```python
from build123d import *

# Parameters (mm, degrees)
BOSS_EXTRUDE1_DEPTH     = 7.5
BOSS_EXTRUDE2_START     = -7.5
SKETCH1_3_W             = 46
SKETCH1_3_H             = 36.5
BOSS_EXTRUDE2_DEPTH     = 5
BOSS_EXTRUDE3_DEPTH     = 2.5
BOSS_EXTRUDE4_DEPTH     = 5
CUT_EXTRUDE1_START      = -5
CUT_EXTRUDE1_DEPTH      = 3
M2_5_CLEARANCE_HOLE1_D  = 2.9
MIRROR1_START           = -16.25
MIRROR1_DEPTH           = 3
MIRROR1_START_2         = -18.25
MIRROR1_2_DEPTH         = 5
MIRROR1_3_OUTLINE_R     = 1.45
MIRROR1_3_DEPTH         = 2
MIRROR1_START_3         = 23
MIRROR1_4_DEPTH         = 2.5
CUT_EXTRUDE2_DEPTH      = 37.094632565
CUT_EXTRUDE2_DEPTH_BACK = 37.094632565
SKETCH10_W              = 15
SKETCH10_H              = 21
CHAMFER1_SIZE           = 5
FILLET1_R               = 1
FILLET2_R               = 1
FILLET6_R               = 1
FILLET7_R               = 1
FILLET8_R               = 1


with BuildPart() as part:
    # Sketch1 → Boss-Extrude1 (new, symmetric)
    with BuildSketch(Plane(origin=(0, 0, 0), x_dir=(1, 0, 0), z_dir=(0, 1, 0))):
        Polygon((23, -18.25), (-23, -18.25), (-23, 18.25), (-25.5, 18.25), (-25.5, -20.75), (25.5, -20.75), (25.5, 18.25), (23, 18.25), align=None)
    extrude(amount=BOSS_EXTRUDE1_DEPTH, both=True)

    # Sketch1<3> → Boss-Extrude2 (add)
    with BuildSketch(Plane(origin=(0, 0, 0), x_dir=(1, 0, 0), z_dir=(0, 1, 0)).offset(BOSS_EXTRUDE2_START)):
        Rectangle(SKETCH1_3_W, SKETCH1_3_H)
    extrude(amount=BOSS_EXTRUDE2_DEPTH)

    # Sketch5 → Boss-Extrude3 (add)
    with BuildSketch(Plane(origin=(-25.5, 32.25, 0), x_dir=(0, 1, 0), z_dir=(-1, 0, 0))):
        Polygon((-47.15, 18.25), (-39.75, 18.25), (-39.75, -20.75), (-47.15, 13.25), align=None)
    extrude(amount=-BOSS_EXTRUDE3_DEPTH)

    # Sketch6 → Boss-Extrude4 (add)
    with BuildSketch(Plane(origin=(0, 0, -18.25), x_dir=(-1, 0, 0), z_dir=(0, 0, -1))):
        Polygon((-12, -10.3), (-14.266838493, -10.3), (-15.883419246, -13.1), (-19.116580754, -13.1), (-20.733161507, -10.3), (-19.116580754, -7.5), (-23, -7.5), (-23, -14.9), (-12, -14.9), align=None)
        Polygon((23, -7.5), (12, -7.5), (12, -10.3), (12, -14.9), (23, -14.9), align=None)
    extrude(amount=-BOSS_EXTRUDE4_DEPTH)

    # Sketch6<3> → Cut-Extrude1 (cut)
    with BuildSketch(Plane(origin=(0, 0, -18.25), x_dir=(-1, 0, 0), z_dir=(0, 0, -1)).offset(CUT_EXTRUDE1_START)):
        Polygon((19.0011107, -7.7), (15.9988893, -7.7), (14.4977786, -10.3), (15.9988893, -12.9), (19.0011107, -12.9), (20.5022214, -10.3), align=None)
    extrude(amount=CUT_EXTRUDE1_DEPTH, mode=Mode.SUBTRACT)

    # M2.5 Clearance Hole1 (through all)
    with Locations(Plane.XY.offset(-16.25)):
        with Locations((-17.5, -10.3), (17.5, -10.3)):
            Hole(M2_5_CLEARANCE_HOLE1_D / 2)

    # Mirror1: read off the stored shape, not the designer's step
    # Mirror1 outline → Mirror1 (cut)
    with BuildSketch(Plane.XY.offset(MIRROR1_START)):
        Polygon((-14.266838493, -10.3), (-15.883419246, -7.5), (-19.116580754, -7.5), (-20.733161507, -10.3), (-19.116580754, -13.1), (-15.883419246, -13.1), align=None)
        Polygon((-15.9988893, -12.9), (-19.0011107, -12.9), (-20.5022214, -10.3), (-19.0011107, -7.7), (-15.9988893, -7.7), (-14.4977786, -10.3), align=None, mode=Mode.SUBTRACT)
    extrude(amount=MIRROR1_DEPTH, mode=Mode.SUBTRACT)

    # Mirror1 2 outline → Mirror1 2 (add)
    with BuildSketch(Plane.XY.offset(MIRROR1_START_2)):
        Polygon((20.733161507, -10.3), (19.116580754, -7.5), (12, -7.5), (12, -10.3), (14.266838493, -10.3), (15.883419246, -13.1), (19.116580754, -13.1), align=None)
        Polygon((15.9988893, -7.7), (19.0011107, -7.7), (20.5022214, -10.3), (19.0011107, -12.9), (15.9988893, -12.9), (14.4977786, -10.3), align=None, mode=Mode.SUBTRACT)
    extrude(amount=MIRROR1_2_DEPTH)

    # Mirror1 3 outline → Mirror1 3 (add)
    with BuildSketch(Plane.XY.offset(MIRROR1_START_2)):
        Polygon((20.5022214, -10.3), (19.0011107, -7.7), (15.9988893, -7.7), (14.4977786, -10.3), (15.9988893, -12.9), (19.0011107, -12.9), align=None)
        with Locations((17.5, -10.3)):
            Circle(MIRROR1_3_OUTLINE_R, mode=Mode.SUBTRACT)
    extrude(amount=MIRROR1_3_DEPTH)

    # Mirror1 4 outline → Mirror1 4 (add)
    with BuildSketch(Plane.YZ.offset(MIRROR1_START_3)):
        Polygon((-14.9, -13.25), (-14.9, -18.25), (-7.5, -18.25), (-7.5, 20.75), align=None)
    extrude(amount=MIRROR1_4_DEPTH)

    # Sketch10 → Cut-Extrude2 (cut, two sides: drawn at the far end of the back side and taken through both)
    with BuildSketch(Plane(origin=(0, 0, 0), x_dir=(1, 0, 0), z_dir=(0, 1, 0)).offset(-CUT_EXTRUDE2_DEPTH_BACK)):
        with Locations((-15.5, 0)):
            Rectangle(SKETCH10_W, SKETCH10_H)
    extrude(amount=CUT_EXTRUDE2_DEPTH + CUT_EXTRUDE2_DEPTH_BACK, mode=Mode.SUBTRACT)

    # Chamfer1
    chamfer1_edges = [part.edges().sort_by_distance(p)[0] for p in [
        (-8, -5, -10.5),
        (-8, -5, 10.5),
    ]]
    chamfer(chamfer1_edges, length=CHAMFER1_SIZE)

    # Fillet1
    fillet1_edges = [part.edges().sort_by_distance(p)[0] for p in [
        (23, 7.5, 0),
        (-23, 2.5, -18.25),
        (-23, 2.5, 18.25),
        (23, 2.5, 18.25),
        (23, 2.5, -18.25),
        (0, 7.5, 18.25),
        (-23, 7.5, 0),
        (-23, -2.5, -14.375),
        (-18, -2.5, -10.5),
        (-23, -5, -10.5),
        (-23, -5, 10.5),
        (-8, -2.5, 0),
        (-18, -2.5, 10.5),
        (-23, -2.5, 14.375),
        (-10.5, -2.5, 8),
        (-10.5, -2.5, -8),
        (0, -2.5, -18.25),
        (0, -2.5, 18.25),
        (23, -2.5, 0),
    ]]
    fillet(fillet1_edges, radius=FILLET1_R)

    # Fillet2
    fillet2_edges = [part.edges().sort_by_distance(p)[0] for p in [
        (25.5, -14.9, -15.75),
        (25.5, -11.2, 3.75),
        (25.5, 0, 20.75),
        (-25.5, 0, 20.75),
        (-25.5, -3.7, -18.25),
        (25.5, -3.7, -18.25),
        (-25.5, 7.5, 1.25),
        (-25.5, -14.9, -15.75),
        (-25.5, -11.2, 3.75),
        (25.5, 7.5, 1.25),
    ]]
    fillet(fillet2_edges, radius=FILLET2_R)

    # Fillet6
    fillet6_edges = [part.edges().sort_by_distance(p)[0] for p in [
        (-12, -14.9, -15.75),
        (12, -14.9, -15.75),
        (12, -11.2, -13.25),
    ]]
    fillet(fillet6_edges, radius=FILLET6_R)

    # Fillet7
    # the kernel refuses this fillet: 1 mm, written as the material it takes off along each edge
    with BuildSketch(Plane(origin=(24.5, 6.5, 19.75), x_dir=(0, 0, 1), z_dir=(0, 1, 0))) as fillet7_piece_1_section:
        Polygon((0, 0), (FILLET7_R, 0), (FILLET7_R, FILLET7_R), (0, FILLET7_R), align=None)
    fillet7_piece_1 = extrude(amount=FILLET7_R, mode=Mode.PRIVATE)
    fillet7_piece_1 = fillet7_piece_1 - Plane(origin=(24.5, 6.5, 19.75), x_dir=(-0.7071067811865476, 0, -0.7071067811865475), z_dir=(0, 1, 0)) * Sphere(FILLET7_R, mode=Mode.PRIVATE)
    add(fillet7_piece_1, mode=Mode.SUBTRACT)
    with BuildSketch(Plane(origin=(-24.5, 6.5, 19.75), x_dir=(0, 0, 1), z_dir=(0, 1, 0))) as fillet7_piece_2_section:
        Polygon((0, 0), (FILLET7_R, 0), (FILLET7_R, -FILLET7_R), (0, -FILLET7_R), align=None)
    fillet7_piece_2 = extrude(amount=FILLET7_R, mode=Mode.PRIVATE)
    fillet7_piece_2 = fillet7_piece_2 - Plane(origin=(-24.5, 6.5, 19.75), x_dir=(0.7071067811865475, 0, -0.7071067811865475), z_dir=(0, 1, 0)) * Sphere(FILLET7_R, mode=Mode.PRIVATE)
    add(fillet7_piece_2, mode=Mode.SUBTRACT)
    with BuildSketch(Plane(origin=(-24.5, 7.5, 20.75), x_dir=(0, 0, -1), z_dir=(1, 0, 0))) as fillet7_piece_3:
        with BuildLine():
            CenterArc((FILLET7_R, -FILLET7_R), FILLET7_R, 90, 90)
            Line((0, -FILLET7_R), (0, 0))
            Line((0, 0), (FILLET7_R, 0))
        make_face()
    extrude(amount=49, mode=Mode.SUBTRACT)

    # Fillet8
    fillet8_edges = [part.edges().sort_by_distance(p)[0] for p in [
        (23, -11.2, 3.75),
        (-23, -11.2, 3.75),
    ]]
    fillet(fillet8_edges, radius=FILLET8_R)


solid = part.part
```
The listing builds one solid part. Answer for the finished solid, in the listing's coordinates (mm). A direction names the side the tool comes from. Coordinates: 2 decimals unless noted, no trailing zeros. Loops run counter-clockwise (first coordinate to the right, second up) from the corner with the lowest first, then second, coordinate; pieces in that order, holes last. Notation, with made-up numbers: M 34,-18.75 L 38,-18.75 A7 cw 38,-6.75 Z; hole C -40,34.25 d7. An arc over 180 degrees is marked long. Answer as CSV lines item,"result". Start each with the question number.
(1) Given pin 1 (1 mm diameter, centred on x = -9, z = -1, fed in from -Y); pin 2 (2 mm diameter, centred on x = 8.5, y = 0, fed in from -Z); pin 3 (4.5 mm diameter, centred on x = -17.5, y = -11.5, fed in from +Z); pin 4 (17 mm diameter, centred on x = -6.5, z = -4, fed in from +Y), each flat-ended and moving along its own axis, determine where each tip first touches the part or whether it passes through.
(2) For faces 5 (the flat face through (-12, -11, -16)), 6 (the flat face through (-19.914, -8.88, -14.771)), 7 (the flat face through (23, 3, 0)), determine the directions among +Z, -Z, +X, -X, +Y, -Y from which every point of the face is accessible in a straight line to the end or side of a thin tool.
(3) The part is cut by section C-C (y = 2). Give the vertices of the cut face in (x, z), and give its area (3 significant figures).
(4) The mould has two halves that part along X. Classify faces 1 (the flat face through (-25.5, -1, 1)), 2 (the flat face through (0, 3, 18.25)), 3 (the cylindrical face through (18.88, -9.86, -17.26)), 4 (the flat face through (24.246, -11.148, 3.988)): pulls with the +X half, pulls with the -X half, needs draft (parallel to the pull), parting line crosses it, or undercut.
(5) The part is cut by section A-A (x = -17.5). Give the vertices of the cut face in (y, z).
(6) Find the intervals of material crossed by L1, parallel to X at y = 6, z = -7; L2, parallel to Z at x = -17, y = -4; L3, parallel to Y at x = -6, z = 8, in increasing order. Write a range as [from, to].
(7) The part is cut by section D-D (x = -4). Give the vertices of the cut face in (y, z), and give its area (3 significant figures).
(8) The part is cut by section B-B (x = 17.5). Give the vertices of the cut face in (y, z).
Determined:
1,pin 1,"through"
1,pin 2,"z = 18.25"
1,pin 3,"z = -13.25"
1,pin 4,"y = -2.5"
2,face 5,"+Z, -Z, -Y"
2,face 6,"+Z"
2,face 7,"-Z, +Y"
3,outline,"M -25.5,-17.25 A1 ccw -24.5,-18.25 L -24,-18.25 A1 ccw -23,-17.25 L -23,17.25 A1 cw -22,18.25 L 22,18.25 A1 cw 23,17.25 L 23,-17.25 A1 ccw 24,-18.25 L 24.5,-18.25 A1 ccw 25.5,-17.25 L 25.5,19.75 A1 ccw 24.5,20.75 L -24.5,20.75 A1 ccw -25.5,19.75 Z"
3,area,"309 mm2"
4,face 1,"pulls with the -X half"
4,face 2,"undercut"
4,face 3,"undercut"
4,face 4,"needs draft"
5,outline,"M -14.9,-18.25 L -11.75,-18.25 L -11.75,-16.25 L -13.1,-16.25 L -13.1,-13.25 L -14.9,-13.25 Z; M -8.85,-18.25 L -3.5,-18.25 A1 ccw -2.5,-17.25 L -2.5,-11.5 A1 ccw -3.5,-10.5 L -7.5,-10.5 L -7.5,-16.25 L -8.85,-16.25 Z; M -7.5,10.5 L -3.5,10.5 A1 ccw -2.5,11.5 L -2.5,17.25 A1 cw -1.5,18.25 L 6.5,18.25 A1 ccw 7.5,19.25 L 7.5,19.75 A1 ccw 6.5,20.75 L -7.5,20.75 Z"
6,L1,"[-25.5, -23], [23, 25.5]"
6,L2,"[-18.25, -10.5], [10.5, 20.75]"
6,L3,"[-7.5, -2.5]"
7,outline,"M -7.5,-18.25 L -3.5,-18.25 A1 ccw -2.5,-17.25 L -2.5,17.25 A1 cw -1.5,18.25 L 6.5,18.25 A1 ccw 7.5,19.25 L 7.5,19.75 A1 ccw 6.5,20.75 L -7.5,20.75 Z"
7,area,"220 mm2"
8,outline,"M -14.9,-18.25 L -11.75,-18.25 L -11.75,-16.25 L -12.9,-16.25 L -12.9,-13.25 L -14.9,-13.25 Z; M -8.85,-18.25 L -3.5,-18.25 A1 ccw -2.5,-17.25 L -2.5,17.25 A1 cw -1.5,18.25 L 6.5,18.25 A1 ccw 7.5,19.25 L 7.5,19.75 A1 ccw 6.5,20.75 L -7.5,20.75 L -7.5,-13.25 L -7.7,-13.25 L -7.7,-16.25 L -8.85,-16.25 Z"
